Source: CAD feature listing. Evaluate the final solid. Frame: model axes, mm. A direction names the side the tool comes from. Coordinates: 2 decimals unless noted, no trailing zeros. Loops run counter-clockwise (first coordinate to the right, second up) from the corner with the lowest first, then second, coordinate; pieces in that order, holes last. Notation, with made-up numbers: M -30.5,86.25 L -26.5,86.25 A12 cw -26.5,106.25 Z; hole C 73,85.25 d6. An arc over 180 degrees is marked long. One line per question, with ' | ' between items. Start each with the question number.
1. Section query B-B, the plane x = -151. Output: boundary loops of the cut face in (y, z).
2. Mould query, pull axis Z, two halves, no side actions, for faces 3 (the cylindrical face through (-98.6, -1.041, 7.932)), 4 (the cylindrical face through (-98.6, 10.161, -4.213)), 5 (the flat face through (-3, 6.25, -7)). Classes: pulls with the +Z half, pulls with the -Z half, needs draft (parallel to the pull), parting line crosses it, or undercut.
3. Access query for faces 1 (the flat face through (0, 9, 0)), 2 (the flat face through (-2, -6.25, 7)). Directions: +Z, -Z, +X, -X, +Y, -Y. A direction counts if a zero-diameter tool reaches every point of the face in a straight line with its end or side. Return the directions, or none.
4. Ray query, probe 1 along X at (y, z) = (0, -9.75); probe 2 along Z at (x, y) = (-96, 0.25). Return the intervals inside material, ascending.
5. Pin query (flat end, axial travel): P1, Ø1.5, axis at x = -24, y = 1, coming from the +Z side; P2, Ø2, axis at x = -3.5, z = -7, coming from the -Y side; P3, Ø5, axis at x = -144.5, y = -3.5, coming from the -Z side; P4, Ø1, axis at y = -5, z = 3.5, coming from the +X side (1 decimal). Return the tip coordinate at first contact, or that it passes through.
6. Section query A-A, the plane z = 0. Output: boundary loops of the cut face in (x, y).
Autodesk Inventor part; units mm, degrees
ref_plane "YZ Plane" through (0, 0, 0) normal (1, 0, 0) x (0, 1, 0)
ref_plane "XZ Plane" through (0, 0, 0) normal (0, 1, 0) x (-1, 0, 0)
ref_plane "XY Plane" through (0, 0, 0) normal (0, 0, 1) x (1, 0, 0)
sketch "スケッチ1" plane through (0, 0, 0) normal (1, 0, 0) x (0, 1, 0)
  circle A0 centre (0, 0) radius 11
  circle A1 centre (0, 0) radius 8
  dimension "d0" = 22
  dimension "d1" = 16
extrude "押し出し1" add sketch "スケッチ1" against normal blind 200
sketch "スケッチ2" plane through (0, 0, 0) normal (0, 0, 1) x (1, 0, 0)
  line L0 (0, 0) -> (0, 6.25)
  line L1 (0, -11) -> (0, 11)
  line L2 (0, 0) -> (0, -6.25)
  line L3 (0, -6.25) -> (-5, -6.25)
  line L4 (-5, -6.25) -> (-5, 6.25)
  line L5 (-5, 6.25) -> (0, 6.25)
  dimension "d4" = 6.25
  dimension "d5" = 6.25
  dimension "d6" = 5
extrude "押し出し2" cut sketch "スケッチ2" along normal mid plane 200
sketch "スケッチ3" plane through (0, 0, 0) normal (0, 0, 1) x (1, 0, 0)
  line L0 (-5, -6.25) -> (-5, 6.25)
  circle A0 centre (-5, 0) radius 6.25
  point P0 (0, 0)
extrude "押し出し3" cut sketch "スケッチ3" along normal mid plane 200 contours A0 L0 picked at (-7.0681, 0.2511)
sketch "スケッチ4" plane through (0, 0, 0) normal (0, 0, 1) x (1, 0, 0)
  circle A0 centre (-190, 0) radius 1.5
  point P0 (0, 0)
  dimension "d11" = 3
extrude "押し出し4" cut sketch "スケッチ4" along normal mid plane 200
thread "ねじ1"
thread "ねじ2"
properties part number "vp16_200" material "PVC 配管"
Taken from the geometry:
1) outline: C 0,0 d22; hole C 0,0 d16
2) face 3: undercut | face 4: parting line crosses it | face 5: needs draft
3) face 1: +Z, -Z, +X, +Y, -Y | face 2: +Z, -Z, +X
4) probe 1: -200 to -191.5, -188.5 to -11.25 | probe 2: -11 to -8, 8 to 11
5) P1: z = 11 | P2: y = -9.22 | P3: z = -10.95 | P4: through
6) outline: M -200,-11 L 0,-11 L 0,-8 L -200,-8 Z; M -200,8 L 0,8 L 0,11 L -200,11 Z
